from build123d import *

# Parameters (mm, degrees)
BOSS_EXTRU_1_DEPTH           = 5
ENL_V_MAT_EXTRU_1_DEPTH      = 112.130553854
ENL_V_MAT_EXTRU_1_DEPTH_BACK = 112.130553854
CONG_1_R                     = 6


with BuildPart() as part:
    # Esquisse1 → Boss.-Extru.1 (new body)
    with BuildSketch(Plane.XY):
        Polygon((0, 0), (65, 0), (65, 90), (18.198511713, 90), (0, 40), align=None)
    extrude(amount=BOSS_EXTRU_1_DEPTH)

    # Esquisse2 → Enlèv. mat.-Extru.1 (cut, two sides: drawn at the far end of the back side and taken through both)
    with BuildSketch(Plane.XY.offset(5).offset(-ENL_V_MAT_EXTRU_1_DEPTH_BACK)):
        Polygon((10.641777725, 40), (25.200587095, 80), (50, 80), (50, 40), align=None)
    extrude(amount=ENL_V_MAT_EXTRU_1_DEPTH + ENL_V_MAT_EXTRU_1_DEPTH_BACK, mode=Mode.SUBTRACT)

    # Congé1
    cong_1_edges = [part.edges().sort_by_distance(p)[0] for p in [
        (50, 40, 2.5),
        (10.641777725, 40, 2.5),
        (25.200587095, 80, 2.5),
        (50, 80, 2.5),
        (0, 40, 2.5),
        (18.198511713, 90, 2.5),
    ]]
    fillet(cong_1_edges, radius=CONG_1_R)


solid = part.part
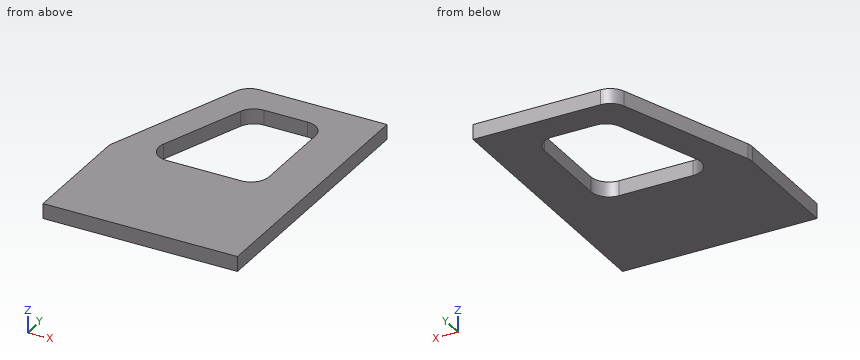
Model file for the job. Use its own axes, mm. Round coordinates to 2 decimals unless told otherwise and drop trailing zeros. Loops run counter-clockwise (first coordinate to the right, second up) from the corner with the lowest first, then second, coordinate; pieces in that order, holes last.
1. Band-saw the part on A-A, the plane x = 34.5. List the corners of the cut face in (y, z), and give its area (3 significant figures).
Check values:
outline: (0, 0) - (40, 0) - (40, 5) - (0, 5) - close; (80, 0) - (90, 0) - (90, 5) - (80, 5) - close
area: 250 mm2
2. Drop a flat-ended pin along its axis: P1, Ø1.5, axis at y = 67, z = 1, coming from the -X side. Give the stop position or say it passes through.
Check values:
P1: stops at x = 9.55
3. Wall check: probe 1 along Y at (x, z) = (41, 2.95); probe 2 along X at (y, z) = (49, 3.35); probe 3 along X at (y, z) = (67, 3.85). Give the ranges that are in metal, low to high.
Check values:
probe 1: y = 0 to 40, 80 to 90
probe 2: x = 3.28 to 13.92, 50 to 65
probe 3: x = 9.83 to 20.47, 50 to 65
4. Band-saw the part on C-C, the plane y = 73. List the corners of the cut face in (x, z).
Check values:
outline: (12.01, 0) - (22.65, 0) - (22.65, 5) - (12.01, 5) - close; (50, 0) - (65, 0) - (65, 5) - (50, 5) - close
5. Band-saw the part on D-D, the plane x = 5.5. List the corners of the cut face in (y, z).
Check values:
outline: (0, 0) - (55.11, 0) - (55.11, 5) - (0, 5) - close
6. Band-saw the part on B-B, the plane z = 3. List the corners of the cut face in (x, y), and give its area (3 significant figures).
Check values:
outline: (0, 0) - (65, 0) - (65, 90) - (22.4, 90) arc R6 ccw to (16.76, 86.05) - (0.36, 40.99) arc R6 ccw to (0, 38.94) - close; hole (13.57, 48.05) arc R6 ccw to (19.21, 40) - (44, 40) arc R6 ccw to (50, 46) - (50, 74) arc R6 ccw to (44, 80) - (29.4, 80) arc R6 ccw to (23.76, 76.05) - close
area: 4,140 mm2
